```python
from build123d import *

# Parameters (mm, degrees)
SKETCH1_W                = 140.9
SKETCH1_H                = 80
PCB_DEPTH                = 1.55
BODYC_DEPTH              = 0.4
BODYC_DEPTH_BACK         = 6.45
SKETCH4_W                = 13.65
SKETCH4_H                = 13.15
BOSS_EXTRUDE4_DEPTH      = 7.1
BOSS_EXTRUDE4_DEPTH_BACK = 1.55
SKETCH5_W                = 4.65
SKETCH5_H                = 3.1
CUT_EXTRUDE3_DEPTH       = 14.1
SKETCH11_W               = 24.15
SKETCH11_H               = 1.55
BOSS_EXTRUDE8_DEPTH      = 29.25
SKETCH7_W                = 24.15
SKETCH7_H                = 1.55
BOSS_EXTRUDE5_DEPTH      = 29.25
CUT_EXTRUDE4_DEPTH       = 89
SKETCH12_R               = 9.15
BATTERY_DEPTH            = 54
SKETCH13_R               = 1
BUTTON_DEPTH             = 1.3
SKETCH14_R               = 1
RESET_DEPTH              = 1.3


with BuildPart() as part:
    # Sketch1 → PCB (new body)
    with BuildSketch(Plane(origin=(0, 0, 0), x_dir=(1, 0, 0), z_dir=(0, 1, 0))):
        Rectangle(SKETCH1_W, SKETCH1_H)
    extrude(amount=PCB_DEPTH)

    # Sketch3 → bodyC (add, two sides)
    with BuildSketch(Plane.ZY.offset(70.45)) as bodyc_sk:
        with BuildLine():
            Line((-34.3, 4.75), (-28.56, 4.75))
            ThreePointArc((-28.56, 4.75), (-26.96, 3.15), (-28.56, 1.55))
            Line((-28.56, 1.55), (-34.3, 1.55))
            ThreePointArc((-34.3, 1.55), (-35.9, 3.15), (-34.3, 4.75))
        make_face()
    extrude(amount=BODYC_DEPTH)
    extrude(bodyc_sk.sketch, amount=-BODYC_DEPTH_BACK)

    # Sketch4 → Boss-Extrude4 (add, two sides)
    with BuildSketch(Plane(origin=(0, 1.55, 0), x_dir=(1, 0, 0), z_dir=(0, 1, 0))) as boss_extrude4_sk:
        with Locations((-68.275, 17.575)):
            Rectangle(SKETCH4_W, SKETCH4_H)
    extrude(amount=BOSS_EXTRUDE4_DEPTH)
    extrude(boss_extrude4_sk.sketch, amount=-BOSS_EXTRUDE4_DEPTH_BACK)

    # Sketch5 → Cut-Extrude3 (cut)
    with BuildSketch(Plane.XY.offset(-11)):
        with Locations((-72.775, 1.55)):
            Rectangle(SKETCH5_W, SKETCH5_H)
    extrude(amount=-CUT_EXTRUDE3_DEPTH, mode=Mode.SUBTRACT)

    # Sketch11 → Boss-Extrude8 (add)
    with BuildSketch(Plane(origin=(0, 1.55, 0), x_dir=(1, 0, 0), z_dir=(0, 1, 0))):
        with Locations((-32.275, 27.625)):
            Rectangle(SKETCH11_W, SKETCH11_H)
    extrude(amount=BOSS_EXTRUDE8_DEPTH)

    # Sketch7 → Boss-Extrude5 (add)
    with BuildSketch(Plane(origin=(0, 1.55, 0), x_dir=(1, 0, 0), z_dir=(0, 1, 0))):
        with Locations((-32.275, -27.325)):
            Rectangle(SKETCH7_W, SKETCH7_H)
    extrude(amount=BOSS_EXTRUDE5_DEPTH)

    # Sketch8 → Cut-Extrude4 (cut)
    with BuildSketch(Plane.XY.offset(28.1)):
        Polygon((-44.35, 30.8), (-20.2, 24.778728731), (-20.2, 30.8), align=None)
    extrude(amount=-CUT_EXTRUDE4_DEPTH, mode=Mode.SUBTRACT)

    # Sketch12 → Battery (add)
    with BuildSketch(Plane.XY.offset(-26.85)):
        with Locations((-32.275, 12.25)):
            Circle(SKETCH12_R)
    extrude(amount=BATTERY_DEPTH)

    # Sketch13 → Button (add)
    with BuildSketch(Plane(origin=(0, 1.55, 0), x_dir=(1, 0, 0), z_dir=(0, 1, 0))):
        with Locations((-62.75, -28.6)):
            Circle(SKETCH13_R)
    extrude(amount=BUTTON_DEPTH)

    # Sketch14 → Reset (add)
    with BuildSketch(Plane(origin=(0, 1.55, 0), x_dir=(1, 0, 0), z_dir=(0, 1, 0))):
        with Locations((-25.75, 9.9)):
            Circle(SKETCH14_R)
    extrude(amount=RESET_DEPTH)


solid = part.part
```
Source: CAD feature listing. Evaluate the final solid. Frame: model axes, mm. A direction names the side the tool comes from. Coordinates: 2 decimals unless noted, no trailing zeros. Write each loop counter-clockwise with the first axis right and the second up, starting at its lowest first coordinate (ties: lowest second). Pieces come first, ordered by that corner, then holes. Notation, with made-up numbers: (0, 17) - (15, 17) arc R28 ccw to (15, 56) - close; hole circle Ø8 at (-22.75, 88.25). An arc over 180 degrees is marked (long way). Answer as a JSON object with one key per item and string values.
Q1. Section query B-B, the plane z = 17.5. Output: boundary loops of the cut face in (x, y) (3 decimals), plus the area to 3 significant figures.
Ans:
{"outline": "(-70.45, 0) - (70.45, 0) - (70.45, 1.55) - (-70.45, 1.55) - close; circle Ø18.3 at (-32.275, 12.25)", "area": "481 mm2"}
Q2. First-contact query: pin 1 Ø1.6 at (y, z) = (4, -32.5) entering from -X; pin 2 Ø6.5 at (x, z) = (-68.5, -19) entering from +Y; pin 3 Ø10 at (y, z) = (20.5, 16.5) entering from -X; pin 4 Ø3 at (x, y) = (-48.5, 4) entering from +Z. Flat tips, straight axial feed; report the tip coordinate or a pass-through.
Ans:
{"pin 1": "stops at x = -70.85", "pin 2": "stops at y = 8.65", "pin 3": "stops at x = -40.83", "pin 4": "passes through"}
Q3. Material intervals for line 1 (Z direction, x = -25, y = 21); line 2 (Y direction, x = 61, z = 35.5); line 3 (Y direction, x = -35.5, z = -21), sorted ascending. Write a range as [from, to].
Ans:
{"line 1": "z = [-28.4, -26.85], [26.55, 28.1]", "line 2": "y = [0, 1.55]", "line 3": "y = [0, 1.55], [3.69, 20.81]"}
Q4. Section query A-A, the plane z = -30. Output: boundary loops of the cut face in (x, y), plus the area to 3 significant figures.
Ans:
{"outline": "(-70.85, 1.55) - (-70.45, 1.55) - (-70.45, 0) - (70.45, 0) - (70.45, 1.55) - (-64, 1.55) - (-64, 4.75) - (-70.85, 4.75) - close", "area": "240 mm2"}
Q5. Set-up query: faces 5 (the cylindrical face through (-41.416, 12.652, -0.524)), 6 (the flat face through (-32, 16, -28.4)), 7 (the flat face through (-68, 8.65, -18)), 8 (the flat face through (-68, 5, -24.15)), 9 (the flat face through (-70.85, 3, -31)). Return all of +Z, -Z, +X, -X, +Y, -Y with unobstructed straight access to the full face (end or side cutting, diameter ignored); none if empty.
Ans:
{"face 5": "none", "face 6": "-Z, +X, +Y", "face 7": "+Z, -Z, -X, +Y", "face 8": "-X, +Y", "face 9": "-Z, -X, +Y, -Y"}
Q6. Section query D-D, the plane x = 53.5. Output: boundary loops of the cut face in (y, z).
Ans:
{"outline": "(0, -40) - (1.55, -40) - (1.55, 40) - (0, 40) - close"}
Q7. Section query C-C, the plane y = 15.5. Output: boundary loops of the cut face in (x, z), plus the area to 3 significant figures.
Ans:
{"outline": "(-44.35, -28.4) - (-20.2, -28.4) - (-20.2, -26.85) - (-23.72, -26.85) - (-23.72, 26.55) - (-20.2, 26.55) - (-20.2, 28.1) - (-44.35, 28.1) - (-44.35, 26.55) - (-40.83, 26.55) - (-40.83, -26.85) - (-44.35, -26.85) - close", "area": "988 mm2"}
Q8. Draft query along X for faces 1 (the flat face through (-64, 3, -31)), 2 (the flat face through (-61.45, 5, -17)), 3 (the flat face through (-70.45, 1, 1)), 4 (the flat face through (-32.44, 27.83, 27.34)). Return one class per face: released by +X, released by -X, zero draft, split by the parting line, or undercut.
Ans:
{"face 1": "undercut", "face 2": "undercut", "face 3": "released by -X", "face 4": "released by +X"}
